from build123d import *

# Parameters (mm, degrees)
SKETCH_1_R          = 20
EXTRUDE_1_DEPTH     = 5
SKETCH_2_R          = 9.7
EXTRUDE_2_DEPTH     = 10
SKETCH_3_R          = 3.5
CUT_EXTRUDE_1_DEPTH = 15
SKETCH_6_R          = 1.5
CUT_EXTRUDE_2_DEPTH = 15
EXTRUDE_3_DEPTH     = 5
SKETCH_13_R         = 1.5
CUT_EXTRUDE_3_DEPTH = 36.661638146


with BuildPart() as part:
    # 草图1 → 凸台-拉伸1 (new body)
    with BuildSketch(Plane(origin=(0, 0, 0), x_dir=(1, 0, 0), z_dir=(0, 1, 0))):
        with Locations(Location((0, 0, 0), (0, 0, 270))):
            Circle(SKETCH_1_R)
    extrude(amount=EXTRUDE_1_DEPTH)

    # 草图2 → 凸台-拉伸2 (add)
    with BuildSketch(Plane(origin=(0, 5, 0), x_dir=(1, 0, 0), z_dir=(0, 1, 0))):
        with Locations(Location((0, 0, 0), (0, 0, 270))):
            Circle(SKETCH_2_R)
    extrude(amount=EXTRUDE_2_DEPTH)

    # 草图3 → 切除-拉伸1 (cut)
    with BuildSketch(Plane(origin=(0, 15, 0), x_dir=(1, 0, 0), z_dir=(0, 1, 0))):
        with Locations(Location((0, 0, 0), (0, 0, 270))):
            Circle(SKETCH_3_R)
    extrude(amount=-CUT_EXTRUDE_1_DEPTH, mode=Mode.SUBTRACT)

    # 草图6 → 切除-拉伸2 (cut)
    with BuildSketch(Plane(origin=(0, 5, 0), x_dir=(1, 0, 0), z_dir=(0, 1, 0))):
        with Locations(Location((-13, 0, 0), (0, 0, 270))):
            Circle(SKETCH_6_R)
        with Locations(Location((0, 13, 0), (0, 0, 270))):
            Circle(SKETCH_6_R)
        with Locations(Location((13, 0, 0), (0, 0, 270))):
            Circle(SKETCH_6_R)
        with Locations(Location((0, -13, 0), (0, 0, 270))):
            Circle(SKETCH_6_R)
    extrude(amount=-CUT_EXTRUDE_2_DEPTH, mode=Mode.SUBTRACT)

    # 草图12 → 凸台-拉伸3 (add)
    with BuildSketch(Plane(origin=(0, 0, 0), x_dir=(1, 0, 0), z_dir=(0, 1, 0))):
        Polygon((-1.255810391, 19.960534569), (0, 22.9), (1.255810391, 19.960534569), (2.870131049, 22.71942666), (3.747626292, 19.645745015), (5.694998416, 22.18055439), (6.180339887, 19.021130326), (8.430052256, 21.291881527), (8.515585831, 18.096541049), (11.032159137, 20.067422973), (10.7165359, 16.88655851), (13.460282277, 18.526489171), (12.748479795, 15.410264856), (15.676128726, 16.693381568), (14.579372548, 13.690942119), (17.64475326, 14.597009365), (16.180339887, 11.755705046), (19.335109494, 12.270433605), (17.526133601, 9.635073482), (20.720539501, 9.750345777), (18.595529718, 7.362491054), (21.779194223, 7.076489171), (19.371663223, 4.973797743), (22.494378042, 4.291032104), (19.842294026, 2.506664671), (22.854812081, 1.437902897), (20, 0), (22.854812081, -1.437902897), (19.842294026, -2.506664671), (22.494378042, -4.291032104), (19.371663223, -4.973797743), (21.779194223, -7.076489171), (18.595529718, -7.362491054), (20.720539501, -9.750345777), (17.526133601, -9.635073482), (19.335109494, -12.270433605), (16.180339887, -11.755705046), (17.64475326, -14.597009365), (14.579372548, -13.690942119), (15.676128726, -16.693381568), (12.748479795, -15.410264856), (13.460282277, -18.526489171), (10.7165359, -16.88655851), (11.032159137, -20.067422973), (8.515585831, -18.096541049), (8.430052256, -21.291881527), (6.180339887, -19.021130326), (5.694998416, -22.18055439), (3.747626292, -19.645745015), (2.870131049, -22.71942666), (1.255810391, -19.960534569), (0, -22.9), (-1.255810391, -19.960534569), (-2.870131049, -22.71942666), (-3.747626292, -19.645745015), (-5.694998416, -22.18055439), (-6.180339887, -19.021130326), (-8.430052256, -21.291881527), (-8.515585831, -18.096541049), (-11.032159137, -20.067422973), (-10.7165359, -16.88655851), (-13.460282277, -18.526489171), (-12.748479795, -15.410264856), (-15.676128726, -16.693381568), (-14.579372548, -13.690942119), (-17.64475326, -14.597009365), (-16.180339887, -11.755705046), (-19.335109494, -12.270433605), (-17.526133601, -9.635073482), (-20.720539501, -9.750345777), (-18.595529718, -7.362491054), (-21.779194223, -7.076489171), (-19.371663223, -4.973797743), (-22.494378042, -4.291032104), (-19.842294026, -2.506664671), (-22.854812081, -1.437902897), (-20, 0), (-22.854812081, 1.437902897), (-19.842294026, 2.506664671), (-22.494378042, 4.291032104), (-19.371663223, 4.973797743), (-21.779194223, 7.076489171), (-18.595529718, 7.362491054), (-20.720539501, 9.750345777), (-17.526133601, 9.635073482), (-19.335109494, 12.270433605), (-16.180339887, 11.755705046), (-17.64475326, 14.597009365), (-14.579372548, 13.690942119), (-15.676128726, 16.693381568), (-12.748479795, 15.410264856), (-13.460282277, 18.526489171), (-10.7165359, 16.88655851), (-11.032159137, 20.067422973), (-8.515585831, 18.096541049), (-8.430052256, 21.291881527), (-6.180339887, 19.021130326), (-5.694998416, 22.18055439), (-3.747626292, 19.645745015), (-2.870131049, 22.71942666), align=None)
    extrude(amount=EXTRUDE_3_DEPTH)

    # 草图13 → 切除-拉伸3 (cut, through all)
    with BuildSketch(Plane(origin=(0, 15, 0), x_dir=(1, 0, 0), z_dir=(0, 1, 0))):
        with Locations(Location((0, 13, 0), (0, 0, 270))):
            Circle(SKETCH_13_R)
        with Locations(Location((13, 0, 0), (0, 0, 270))):
            Circle(SKETCH_13_R)
        with Locations(Location((0, -13, 0), (0, 0, 270))):
            Circle(SKETCH_13_R)
        with Locations(Location((-13, 0, 0), (0, 0, 270))):
            Circle(SKETCH_13_R)
    extrude(amount=-CUT_EXTRUDE_3_DEPTH, mode=Mode.SUBTRACT)


solid = part.part
Input: part model. Units: mm. Frame: model coordinates. A direction names the side the tool comes from. Coordinates: 2 decimals unless noted, no trailing zeros. Loops run counter-clockwise (first coordinate to the right, second up) from the corner with the lowest first, then second, coordinate; pieces in that order, holes last.
Q1. Cut plane A-A (y = 9.5). Output: boundary loops of the cut face in (x, z), then the cut area to 3 significant figures.
Q2. Material intervals for line 1 (X direction, y = 10.5, z = 0); line 2 (Y direction, x = 10, z = 2); line 3 (X direction, y = 1, z = 21.5), sorted ascending.
Q3. Set-up query: faces 4 (the face through (20.17, 2.46, -7.22)), 5 (the face through (-16.902, 2.465, -13.156)), 6 (the face through (-5.94, 2.46, -20.58)). Return all of +Z, -Z, +X, -X, +Y, -Y with unobstructed straight access to the full face (end or side cutting, diameter ignored); none if empty.
Q4. Cut plane C-C (x = 5). Output: boundary loops of the cut face in (y, z).
Q5. Draft query along X for faces 1 (the face through (5.94, 2.46, 20.58)), 2 (the face through (20.95, 2.46, 4.63)), 3 (the face through (-19.643, 2.465, -8.54)). Return one class per face: +X half, -X half, draft (parallel to the pull), parting line (faces both ways), or undercut.
Q6. Cut plane D-D (y = 3). Give the number of separate pieces and of enclosed holes in the cut face, then the cut area to 3 significant figures.
Q7. Contact query for flat-ended pins moving along their axis: pin 1 (8 mm diameter, centred on x = 3.5, y = 7.5, fed in from -Z); pin 2 (7.5 mm diameter, centred on x = 1.5, z = 0.5, fed in from +Y); pin 3 (1 mm diameter, centred on y = 12, z = 6.5, fed in from -X); pin 4 (6.5 mm diameter, centred on x = 0, z = 0, fed in from +Y). Output: stop coordinate, or through.
Q8. Cut plane B-B (z = 13). Output: boundary loops of the cut face in (x, y), then the cut area to 3 significant figures.
Working result:
1. outline: circle Ø19.4 at (0, 0); hole circle Ø7 at (0, 0)
1. area: 257 mm2
2. line 1: x = -9.7 to -3.5, 3.5 to 9.7
2. line 2: y = 0 to 5
2. line 3: x = -5.8 to -5.17, -3.22 to -2.16, -0.6 to 0.6, 2.16 to 3.22, 5.17 to 5.8
3. face 4: +X, +Y, -Y
3. face 5: +Y, -Y
3. face 6: -Z, +Y, -Y
4. outline: (0, -21.28) - (5, -21.28) - (5, -8.31) - (15, -8.31) - (15, 8.31) - (5, 8.31) - (5, 21.28) - (0, 21.28) - close
5. face 1: undercut
5. face 2: +X half
5. face 3: -X half
6. separate pieces: 1
6. enclosed holes: 4
6. area: 1,410 mm2
7. pin 1: stops at z = -22.72
7. pin 2: stops at y = 15
7. pin 3: stops at x = -7.62
7. pin 4: stops at y = 5
8. outline: (-16.82, 0) - (-1.5, 0) - (-1.5, 5) - (-16.82, 5) - close; (1.5, 0) - (16.82, 0) - (16.82, 5) - (1.5, 5) - close
8. area: 153 mm2
